```python
from build123d import *

# Parameters (mm, degrees)
BOSS_EXTRUDE1_DEPTH                      = 8
F_4_4_4_4_DIAMETER_HOLE1_D               = 4.4
F_4_4_4_4_DIAMETER_HOLE1_DEPTH           = 6
F_4_4_4_4_DIAMETER_HOLE1_TIP             = 2.2
F_4_4_4_4_DIAMETER_HOLE1_ON_FACE_2_D     = 4.4
F_4_4_4_4_DIAMETER_HOLE1_ON_FACE_2_DEPTH = 6
F_4_4_4_4_DIAMETER_HOLE1_ON_FACE_2_TIP   = 2.2
F_3_4_START                              = 6.4999999
F_3_4_3_4_DIAMETER_HOLE1_OUTLINE_R       = 1.7
F_3_4_3_4_DIAMETER_HOLE1_DEPTH           = 1.5000001
F_3_4_3_4_DIAMETER_HOLE1_2_OUTLINE_R     = 1.7
F_3_4_3_4_DIAMETER_HOLE1_2_DEPTH         = 1.5000001
FILLET1_R                                = 0.5


# Read off the part's stored shape, not the designer's step: Ø3.4 (3.4) Diameter Hole1
with BuildPart() as part:
    # Sketch1 → Boss-Extrude1 (new body)
    with BuildSketch(Plane.XY):
        Polygon((-12, 0), (12, 0), (12, 8), (4, 8), (4, 16), (-4, 16), (-4, 8), (-12, 8), align=None)
    extrude(amount=BOSS_EXTRUDE1_DEPTH)

    # Ø4.4 (4.4) Diameter Hole1
    with Locations(Plane(origin=(0, 4, 8), x_dir=(1, 0, 0), z_dir=(0, 0, 1))):
        with Locations((0, 0), (0, 8)):
            Hole(F_4_4_4_4_DIAMETER_HOLE1_D / 2, depth=F_4_4_4_4_DIAMETER_HOLE1_DEPTH)
            with Locations((0, 0, -(F_4_4_4_4_DIAMETER_HOLE1_DEPTH + F_4_4_4_4_DIAMETER_HOLE1_TIP / 2))):  # 90° drill point
                Cone(0, F_4_4_4_4_DIAMETER_HOLE1_D / 2, F_4_4_4_4_DIAMETER_HOLE1_TIP, mode=Mode.SUBTRACT)

    # Ø4.4 (4.4) Diameter Hole1 on face 2
    with Locations(Plane(origin=(8, 0, 4), x_dir=(0, 0, -1), z_dir=(0, -1, 0))):
        with Locations((0, 0), (0, -16)):
            Hole(F_4_4_4_4_DIAMETER_HOLE1_ON_FACE_2_D / 2, depth=F_4_4_4_4_DIAMETER_HOLE1_ON_FACE_2_DEPTH)
            with Locations((0, 0, -(F_4_4_4_4_DIAMETER_HOLE1_ON_FACE_2_DEPTH + F_4_4_4_4_DIAMETER_HOLE1_ON_FACE_2_TIP / 2))):  # 90° drill point
                Cone(0, F_4_4_4_4_DIAMETER_HOLE1_ON_FACE_2_D / 2, F_4_4_4_4_DIAMETER_HOLE1_ON_FACE_2_TIP, mode=Mode.SUBTRACT)

    # Ø3.4 (3.4) Diameter Hole1 outline → Ø3.4 (3.4) Diameter Hole1 (cut)
    with BuildSketch(Plane(origin=(0, 0, 0), x_dir=(1, 0, 0), z_dir=(0, 1, 0)).offset(F_3_4_START)):
        with Locations((-8, -4)):
            Circle(F_3_4_3_4_DIAMETER_HOLE1_OUTLINE_R)
        with Locations((8, -4)):
            Circle(F_3_4_3_4_DIAMETER_HOLE1_OUTLINE_R)
    extrude(amount=F_3_4_3_4_DIAMETER_HOLE1_DEPTH, mode=Mode.SUBTRACT)

    # 3.4 _3.4_ Diameter Hole1 2 outline → 3.4 _3.4_ Diameter Hole1 2 (cut)
    with BuildSketch(Plane.XY):
        with Locations((0, 4)):
            Circle(F_3_4_3_4_DIAMETER_HOLE1_2_OUTLINE_R)
        with Locations((0, 12)):
            Circle(F_3_4_3_4_DIAMETER_HOLE1_2_OUTLINE_R)
    extrude(amount=F_3_4_3_4_DIAMETER_HOLE1_2_DEPTH, mode=Mode.SUBTRACT)

    # Fillet1
    fillet1_edges = [part.edges().sort_by_distance(p)[0] for p in [
        (8, 8, 0),
        (12, 4, 0),
        (0, 0, 0),
        (-12, 4, 0),
        (12, 4, 8),
        (-12, 8, 4),
        (-4, 8, 4),
        (-4, 16, 4),
        (4, 16, 4),
        (4, 8, 4),
        (12, 8, 4),
        (12, 0, 4),
        (-12, 0, 4),
        (8, 8, 8),
        (4, 12, 8),
        (0, 16, 8),
        (-4, 12, 8),
        (-8, 8, 8),
        (-12, 4, 8),
        (-8, 8, 0),
        (0, 0, 8),
        (-4, 12, 0),
        (0, 16, 0),
        (4, 12, 0),
    ]]
    fillet(fillet1_edges, radius=FILLET1_R)


solid = part.part
```
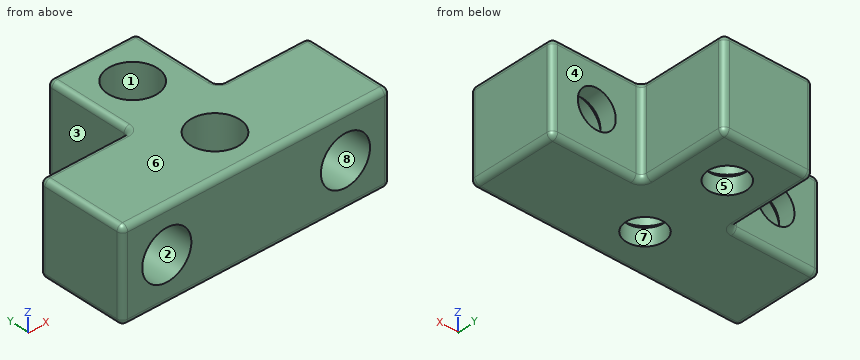
Input: part model. Units: mm. Frame: model coordinates. Face numbers are marked on the shaded views. A direction names the side the tool comes from. Round coordinates to 2 decimals unless told otherwise and drop trailing zeros. Loops run counter-clockwise (first coordinate to the right, second up) from the corner with the lowest first, then second, coordinate; pieces in that order, holes last. Notation, with made-up numbers: M -9,2 L 21,2 A23 ccw 21,26 Z; hole C 7.5,42.5 d5. An arc over 180 degrees is marked long. Answer in a Markdown table with one row per item. Add a question column.
1. Set-up query: the marked faces 1, 2, 3, 4 and 5. Return all of +Z, -Z, +X, -X, +Y, -Y with unobstructed straight access to the full face (end or side cutting, diameter ignored); none if empty.
2. Section A-A (y = 4). Output: boundary loops of the cut face in (x, z), and give its area (3 significant figures).
3. Ray query, probe 1 along Y at (x, z) = (0, 6.8); probe 2 along X at (y, z) = (4, 6.5); probe 3 along X at (y, z) = (3.5, 4.5). Return the intervals inside material, ascending.
4. Section B-B (z = 4). Give the number of separate pieces and of enclosed holes in the cut face, and give its area (3 significant figures).
5. Contact query for flat-ended pins moving along their axis: pin 1 (3 mm diameter, centred on x = 8, z = 4, fed in from -Y); pin 2 (4 mm diameter, centred on x = -6, z = 3, fed in from -Y); pin 3 (4 mm diameter, centred on x = -8, z = 4, fed in from -Y); pin 4 (3.5 mm diameter, centred on y = 12, z = 2.5, fed in from -X). Output: stop coordinate, or through.
6. Mould query, pull axis Z, two halves, no side actions, for the marked faces 6, 7 and 8. Classes: released by +Z, released by -Z, zero draft, split by the parting line, or undercut.
7. Section C-C (x = -8). Output: boundary loops of the cut face in (y, z).
8. Section D-D (y = 12). Output: boundary loops of the cut face in (x, z).
Values follow:
| question | item | result |
|---|---|---|
| 1 | face 1 | +Z |
| 1 | face 2 | -Y |
| 1 | face 3 | +Z, -Z, -X, +Y |
| 1 | face 4 | +Z, -Z, +X, +Y |
| 1 | face 5 | +Z, -Z |
| 2 | outline | M -12,0.5 A0.5 ccw -11.5,0 L -1.7,0 L -1.7,1.5 L -2.2,2 L -2.2,8 L -11.5,8 A0.5 ccw -12,7.5 Z; M 1.7,0 L 11.5,0 A0.5 ccw 12,0.5 L 12,7.5 A0.5 ccw 11.5,8 L 2.2,8 L 2.2,2 L 1.7,1.5 Z; hole C -8,4 d4.4; hole C 8,4 d4.4 |
| 2 | area | 128 mm^2 |
| 3 | probe 1 | 0 to 1.8, 6.2 to 9.8, 14.2 to 16 |
| 3 | probe 2 | -12 to -2.2, 2.2 to 12 |
| 3 | probe 3 | -12 to -10.14, -5.86 to -2.14, 2.14 to 5.86, 10.14 to 12 |
| 4 | separate pieces | 3 |
| 4 | enclosed holes | 2 |
| 4 | area | 158 mm^2 |
| 5 | pin 1 | through |
| 5 | pin 2 | y = 0 |
| 5 | pin 3 | y = 6.2 |
| 5 | pin 4 | x = -4 |
| 6 | face 6 | released by +Z |
| 6 | face 7 | zero draft |
| 6 | face 8 | undercut |
| 7 | outline | M 0,0.5 A0.5 ccw 0.5,0 L 7.5,0 A0.5 ccw 8,0.5 L 8,2.3 L 6.5,2.3 L 6,1.8 L 0,1.8 Z; M 0,6.2 L 6,6.2 L 6.5,5.7 L 8,5.7 L 8,7.5 A0.5 ccw 7.5,8 L 0.5,8 A0.5 ccw 0,7.5 Z |
| 8 | outline | M -4,0.5 A0.5 ccw -3.5,0 L -1.7,0 L -1.7,1.5 L -2.2,2 L -2.2,8 L -3.5,8 A0.5 ccw -4,7.5 Z; M 1.7,0 L 3.5,0 A0.5 ccw 4,0.5 L 4,7.5 A0.5 ccw 3.5,8 L 2.2,8 L 2.2,2 L 1.7,1.5 Z |
